Check sheet for the modelled part. Datum: model origin and axes. Units: mm. Give positions to 0.01 mm unless a question says otherwise; leave off trailing zeros. Answer as a JSON object with one key per item and string values.
from build123d import *

# Parameters (mm, degrees)
SKETCH1_W            = 114.3
SKETCH1_H            = 1219.2
BASE_EXTRUDE_DEPTH   = 38.1
CUT_EXTRUDE1_DEPTH   = 1220.2
MIRROR2_COPY_1_DEPTH = 1220.2
MIRROR2_COPY_2_DEPTH = 1220.2


with BuildPart() as part:
    # Sketch1 → Base Extrude (new body)
    with BuildSketch(Plane(origin=(0, 0, 0), x_dir=(1, 0, 0), z_dir=(0, 1, 0))):
        Rectangle(SKETCH1_W, SKETCH1_H)
    extrude(amount=BASE_EXTRUDE_DEPTH)

    # Sketch3 → Cut-Extrude1 (cut, through all)
    with BuildSketch(Plane.XY.offset(609.6)):
        Polygon((-42.06875, 38.1), (-34.13125, 38.1), (-34.13125, 34.13125), (-28.347265172, 34.13125), (-34.13125, 25.49525), (-42.06875, 25.49525), (-47.397265172, 34.13125), (-42.06875, 34.13125), align=None)
        Polygon((-23.01875, 28.347265172), (-23.01875, 23.01875), (-19.05, 23.01875), (-19.05, 15.08125), (-23.01875, 15.08125), (-23.01875, 9.297265172), (-31.65475, 15.08125), (-31.65475, 23.01875), align=None)
        Polygon((-28.802734828, 3.96875), (-34.13125, 3.96875), (-34.13125, 0), (-42.06875, 0), (-42.06875, 3.96875), (-47.852734828, 3.96875), (-42.06875, 12.60475), (-34.13125, 12.60475), align=None)
        Polygon((-53.18125, 9.752734828), (-53.18125, 15.08125), (-57.15, 15.08125), (-57.15, 23.01875), (-53.18125, 23.01875), (-53.18125, 28.802734828), (-44.54525, 23.01875), (-44.54525, 15.08125), align=None)
    cut_extrude1 = extrude(amount=-CUT_EXTRUDE1_DEPTH, mode=Mode.SUBTRACT)

    # Mirror1: Cut-Extrude1 across plane
    add(cut_extrude1.mirror(Plane.ZY.offset(19.05)), mode=Mode.SUBTRACT)

    # Mirror2 copy 1 sketch → Mirror2 copy 1 (cut, through all)
    with BuildSketch(Plane(origin=(76.3905, 0, 609.6), x_dir=(1, 0, 0), z_dir=(0, 0, 1))):
        Polygon((-42.06875, 38.1), (-34.13125, 38.1), (-34.13125, 34.13125), (-28.347265172, 34.13125), (-34.13125, 25.49525), (-42.06875, 25.49525), (-47.397265172, 34.13125), (-42.06875, 34.13125), align=None)
        Polygon((-23.01875, 28.347265172), (-23.01875, 23.01875), (-19.05, 23.01875), (-19.05, 15.08125), (-23.01875, 15.08125), (-23.01875, 9.297265172), (-31.65475, 15.08125), (-31.65475, 23.01875), align=None)
        Polygon((-28.802734828, 3.96875), (-34.13125, 3.96875), (-34.13125, 0), (-42.06875, 0), (-42.06875, 3.96875), (-47.852734828, 3.96875), (-42.06875, 12.60475), (-34.13125, 12.60475), align=None)
        Polygon((-53.18125, 9.752734828), (-53.18125, 15.08125), (-57.15, 15.08125), (-57.15, 23.01875), (-53.18125, 23.01875), (-53.18125, 28.802734828), (-44.54525, 23.01875), (-44.54525, 15.08125), align=None)
    extrude(amount=-MIRROR2_COPY_1_DEPTH, mode=Mode.SUBTRACT)

    # Mirror2 copy 2 sketch → Mirror2 copy 2 (cut, through all)
    with BuildSketch(Plane(origin=(38.2905, 0, 609.6), x_dir=(-1, 0, 0), z_dir=(0, 0, 1))):
        Polygon((-42.06875, -38.1), (-34.13125, -38.1), (-34.13125, -34.13125), (-28.347265172, -34.13125), (-34.13125, -25.49525), (-42.06875, -25.49525), (-47.397265172, -34.13125), (-42.06875, -34.13125), align=None)
        Polygon((-23.01875, -28.347265172), (-23.01875, -23.01875), (-19.05, -23.01875), (-19.05, -15.08125), (-23.01875, -15.08125), (-23.01875, -9.297265172), (-31.65475, -15.08125), (-31.65475, -23.01875), align=None)
        Polygon((-28.802734828, -3.96875), (-34.13125, -3.96875), (-34.13125, 0), (-42.06875, 0), (-42.06875, -3.96875), (-47.852734828, -3.96875), (-42.06875, -12.60475), (-34.13125, -12.60475), align=None)
        Polygon((-53.18125, -9.752734828), (-53.18125, -15.08125), (-57.15, -15.08125), (-57.15, -23.01875), (-53.18125, -23.01875), (-53.18125, -28.802734828), (-44.54525, -23.01875), (-44.54525, -15.08125), align=None)
    extrude(amount=-MIRROR2_COPY_2_DEPTH, mode=Mode.SUBTRACT)


solid = part.part
1. Scan lines: L1, parallel to X at y = 18, z = 64; L2, parallel to Y at x = 32.5, z = -459; L3, parallel to Y at x = 4, z = 268. Record each from-to range of solid material in increasing order. Write a range as [from, to].
Determined:
{"L1": "[-44.55, -31.65], [-6.45, 6.45], [19.05, 19.24], [31.85, 44.74]", "L2": "[0, 3.97], [9.88, 28.45], [34.13, 38.1]", "L3": "[0, 3.97], [12.56, 25.55], [34.13, 38.1]"}
2. Sectioned sample at A-A, the plane z = 27.5. State how many separate pieces and enclosed holes the cut face has, plus the area to 3 significant figures.
Determined:
{"separate pieces": "1", "enclosed holes": "3", "area": "2,580 mm^2"}
3. Go/stop test with flat-tipped pins: P1, Ø2.5, axis at y = 18, z = 210.5, coming from the +X side; P2, Ø1, axis at x = -37.5, z = -28, coming from the -Y side. Record where each tip stops, or that it passes through.
Determined:
{"P1": "x = 44.74", "P2": "y = 12.6"}
